CAD build for the part. Positions are in the model's coordinates, mm. A direction names the side the tool comes from. Round coordinates to 2 decimals unless told otherwise and drop trailing zeros. Loops run counter-clockwise (first coordinate to the right, second up) from the corner with the lowest first, then second, coordinate; pieces in that order, holes last. Notation, with made-up numbers: M 80,78 L 94,78 A19 ccw 94,115 Z; hole C 43.5,-11 d8. An arc over 180 degrees is marked long. Use a Markdown table: item, result. Add a question column.
(1) Band-saw the part on C-C, the plane z = 45.17. Write the cut outline in (x, y).
(2) Band-saw the part on B-B, the plane x = 6. Write the cut outline in (y, z).
(3) Band-saw the part on D-D, the plane y = -48. Write the cut outline in (x, z).
(4) Which spindle directions (+Z, -Z, +X, -X, +Y, -Y) get a long thin tool onto all of the face, cutting with end or side? Do faces 1 (the face through (4.357, -21.158, -26.803)), 2 (the face through (4.87, 0, 25)), 3 (the face through (6, -41, -10.65)), 4 (the face through (6, 21, -10.65)), 5 (the face through (12.87, -11, -14)). Say none if no direction does.
(5) Flat gauge pins, fed straight in: P1, Ø6.5, axis at x = 6, z = 39.5, coming from the -Y side; P2, Ø2, axis at x = 7, y = -3, coming from the -Z side; P3, Ø5, axis at x = 7.5, z = 4, coming from the +Y side. Where does each tip first touch, or does it go through?
(6) Two-plate mould, pull along Y, no slides. Class faces 6 (the face through (6, 0, 51.17)), 7 (the face through (4, -11.852, 35)), 8 (the face through (6.279, 0.132, 42.173)): released by +Y, released by -Y, zero draft, split by the parting line, or undercut.
(7) Wall check: L1, parallel to Y at x = 3.5, z = 0; L2, parallel to Z at x = 6.5, y = 0.5; L3, parallel to Y at x = 4.25, z = 45.17. Give the ranges that are in metal, low to high.
(8) Band-saw the part on A-A, the plane y = 0. Write the cut outline in (x, z), and give its area (3 significant figures).
from build123d import *

# Parameters (mm, degrees)
SKETCH1_W                       = 21.3
SKETCH1_H                       = 29
BOSS_EXTRUDE1_DEPTH             = 25.87
CUT_EXTRUDE1_DEPTH              = 32.510782282
SKETCH5_W                       = 5
SKETCH5_H                       = 23.7
BOSS_EXTRUDE2_DEPTH             = 31.52
SKETCH6_W                       = 5
SKETCH6_H                       = 23.7
BOSS_EXTRUDE3_DEPTH             = 15.9
SKETCH7_W                       = 25.87
SKETCH7_H                       = 94
BOSS_EXTRUDE4_DEPTH             = 20
CUT_EXTRUDE2_DEPTH              = 107.224130027
SKETCH10_W                      = 25.87
SKETCH10_H                      = 23.7
BOSS_EXTRUDE5_DEPTH             = 9
SKETCH13_W                      = 25.74
SKETCH13_H                      = 140
CUT_EXTRUDE3_DEPTH              = 109.61791657
SKETCH14_W                      = 7
SKETCH14_H                      = 23.7
BOSS_EXTRUDE6_DEPTH             = 8
F_6_0MM_CLEARANCE_DOWEL_HOLE1_D = 6


with BuildPart() as part:
    # Sketch1 → Boss-Extrude1 (new body)
    with BuildSketch(Plane(origin=(0, 0, 0), x_dir=(0, 0, -1), z_dir=(1, 0, 0))):
        Rectangle(SKETCH1_W, SKETCH1_H)
    boss_extrude1 = extrude(amount=BOSS_EXTRUDE1_DEPTH)

    # Sketch3 → Cut-Extrude1 (cut, through all)
    with BuildSketch(Plane(origin=(25.87, 0, 0), x_dir=(0, 0, -1), z_dir=(1, 0, 0))):
        Polygon((-7.998349571, -14.5), (-10.65, -11.848349571), (-10.65, -14.5), align=None)
        Polygon((-10.65, 11.848349571), (-10.65, 14.5), (-7.998349571, 14.5), align=None)
    cut_extrude1 = extrude(amount=-CUT_EXTRUDE1_DEPTH, mode=Mode.SUBTRACT)

    # Sketch5 → Boss-Extrude2 (add)
    with BuildSketch(Plane.XY.offset(10.65)):
        with Locations((23.37, -0.001650429)):
            Rectangle(SKETCH5_W, SKETCH5_H)
        with Locations((2.5, -0.001650429)):
            Rectangle(SKETCH5_W, SKETCH5_H)
    boss_extrude2 = extrude(amount=BOSS_EXTRUDE2_DEPTH)

    # Sketch6 → Boss-Extrude3 (add)
    with BuildSketch(Plane.ZY.offset(-20.87)):
        with Locations((39.67, -0.001650429)):
            Rectangle(SKETCH6_W, SKETCH6_H)
    extrude(amount=BOSS_EXTRUDE3_DEPTH)

    # Sketch7 → Boss-Extrude4 (add)
    with BuildSketch(Plane(origin=(0, 0, -10.65), x_dir=(-1, 0, 0), z_dir=(0, 0, -1))):
        with Locations((-12.935, -20.5)):
            Rectangle(SKETCH7_W, SKETCH7_H)
    boss_extrude4 = extrude(amount=BOSS_EXTRUDE4_DEPTH)

    # Sketch9 → Cut-Extrude2 (cut, through all)
    with BuildSketch(Plane(origin=(0, -67.5, 0), x_dir=(-1, 0, 0), z_dir=(0, -1, 0))):
        with BuildLine():
            ThreePointArc((-26.12, 16.65), (-12.87, 29.9), (0.38, 16.65))
            Line((0.38, 16.65), (0.38, 30.65))
            Line((0.38, 30.65), (-26.12, 30.65))
            Line((-26.12, 30.65), (-26.12, 16.65))
        make_face()
    cut_extrude2 = extrude(amount=-CUT_EXTRUDE2_DEPTH, mode=Mode.SUBTRACT)

    # Sketch10 → Boss-Extrude5 (add)
    with BuildSketch(Plane.XY.offset(42.17)):
        with Locations((12.935, -0.001650429)):
            Rectangle(SKETCH10_W, SKETCH10_H)
    boss_extrude5 = extrude(amount=BOSS_EXTRUDE5_DEPTH)

    # Sketch13 → Cut-Extrude3 (cut, through all)
    with BuildSketch(Plane.XY.offset(51.17)):
        with Locations((0, -0.001650429)):
            Rectangle(SKETCH13_W, SKETCH13_H)
    cut_extrude3 = extrude(amount=-CUT_EXTRUDE3_DEPTH, mode=Mode.SUBTRACT)

    # Mirror2: Boss-Extrude1, Cut-Extrude1, Boss-Extrude2, Boss-Extrude4, Cut-Extrude2, Boss-Extrude5, Cut-Extrude3 across plane
    add(boss_extrude1.mirror(Plane(origin=(12.87, 69.998349571, -29.9), x_dir=(0, 0, 1), z_dir=(1, 0, 0))))
    add(cut_extrude1.mirror(Plane(origin=(12.87, 69.998349571, -29.9), x_dir=(0, 0, 1), z_dir=(1, 0, 0))), mode=Mode.SUBTRACT)
    add(boss_extrude2.mirror(Plane(origin=(12.87, 69.998349571, -29.9), x_dir=(0, 0, 1), z_dir=(1, 0, 0))))
    add(boss_extrude4.mirror(Plane(origin=(12.87, 69.998349571, -29.9), x_dir=(0, 0, 1), z_dir=(1, 0, 0))))
    add(cut_extrude2.mirror(Plane(origin=(12.87, 69.998349571, -29.9), x_dir=(0, 0, 1), z_dir=(1, 0, 0))), mode=Mode.SUBTRACT)
    add(boss_extrude5.mirror(Plane(origin=(12.87, 69.998349571, -29.9), x_dir=(0, 0, 1), z_dir=(1, 0, 0))))
    add(cut_extrude3.mirror(Plane(origin=(12.87, 69.998349571, -29.9), x_dir=(0, 0, 1), z_dir=(1, 0, 0))), mode=Mode.SUBTRACT)

    # Sketch14 → Boss-Extrude6 (add)
    with BuildSketch(Plane(origin=(4.87, 0, 0), x_dir=(0, 0, -1), z_dir=(1, 0, 0))):
        with Locations((-42.67, -0.001650429)):
            Rectangle(SKETCH14_W, SKETCH14_H)
    extrude(amount=BOSS_EXTRUDE6_DEPTH)

    # Ø6.0mm Clearance Dowel Hole1 (through all)
    with Locations(Plane(origin=(12.87, 0, 0), x_dir=(0, 0, -1), z_dir=(1, 0, 0))):
        with Locations((-45.17, 0), (0, 0)):
            Hole(F_6_0MM_CLEARANCE_DOWEL_HOLE1_D / 2)


solid = part.part
Return value:
| question | item | result |
|---|---|---|
| 1 | outline | M -0.13,-11.85 L 12.87,-11.85 L 12.87,-3 L -0.13,-3 Z; M -0.13,3 L 12.87,3 L 12.87,11.85 L -0.13,11.85 Z |
| 2 | outline | M -67.5,-27.98 L 26.5,-27.98 L 26.5,-10.65 L 14.5,-10.65 L 14.5,8 L 11.85,10.65 L -11.85,10.65 L -14.5,8 L -14.5,-10.65 L -67.5,-10.65 Z; M -11.85,39.17 L 11.85,39.17 L 11.85,51.17 L -11.85,51.17 Z; hole C 0,0 d6; hole C 0,45.17 d6 |
| 3 | outline | M -0.13,-19.21 A13.25 ccw 12.87,-29.9 L 12.87,-10.65 L -0.13,-10.65 Z |
| 4 | face 1 | -Z, -X, +Y, -Y |
| 4 | face 2 | +X, +Y, -Y |
| 4 | face 3 | +Z, +X, -X, -Y |
| 4 | face 4 | +Z, +X, -X, +Y |
| 4 | face 5 | +Z, -Z, +X, +Y, -Y |
| 5 | P1 | y = -11.85 |
| 5 | P2 | z = -28.97 |
| 5 | P3 | y = 14.5 |
| 6 | face 6 | zero draft |
| 6 | face 7 | released by -Y |
| 6 | face 8 | undercut |
| 7 | L1 | -14.5 to -3, 3 to 14.5 |
| 7 | L2 | -28.27 to -2.96, 2.96 to 10.65, 39.17 to 42.21, 48.13 to 51.17 |
| 7 | L3 | -11.85 to -3, 3 to 11.85 |
| 8 | outline | M -0.13,-19.21 A13.25 ccw 12.87,-29.9 L 12.87,-3 L -0.13,-3 Z; M -0.13,3 L 12.87,3 L 12.87,10.65 L 4.87,10.65 L 4.87,39.17 L 12.87,39.17 L 12.87,42.17 L -0.13,42.17 Z; M -0.13,48.17 L 12.87,48.17 L 12.87,51.17 L -0.13,51.17 Z |
| 8 | area | 635 mm^2 |
